Work out the finished part from the listing and answer in its coordinate system (mm). A direction names the side the tool comes from. Coordinates: 2 decimals unless noted, no trailing zeros. Order: outer loops, then holes, each group sorted by start corner. A loop starts at its lowest first (then second) coordinate and runs counter-clockwise, first axis right, second up.
1. A tool of negligible diameter and unlimited length cuts with its end or side. For faces 4 (the flat face through (29, 10.922, 2)), 5 (the flat face through (1.868, 3.297, -0.626)), 6 (the cylindrical face through (-24.159, 2.352, -3.858)), 7 (the flat face through (-19.553, 13.426, 4.948)), 8 (the flat face through (2.5, -4.4, 1.7)), from which of +Z, -Z, +X, -X, +Y, -Y can it reach the whole face along a straight path? Write none if from no direction.
2. The part is cut by section C-C, the plane y = 9.75. Give the vertices of the cut face in (x, z).
3. The part is cut by section B-B, the plane z = 1.75. Give the vertices of the cut face in (x, y).
4. The part is cut by section A-A, the plane y = 1.25. Give the vertices of the cut face in (x, z).
5. Determine the mould class of faces 1 (the flat face through (-5.059, 0, 2)), 2 (the flat face through (-1, 16.002, -1)), 3 (the cylindrical face through (-29.829, 13.498, 4.465)) for opening direction X: +X half, -X half, draft (parallel to the pull), parting line (faces both ways), or undercut.
6. Flat-ended cylindrical pins translate along their axes: pin 1 Ø12 at (x, y) = (17, 8) entering from -Z; pin 2 Ø5 at (x, z) = (1, -2) entering from +Y; pin 3 Ø4 at (x, z) = (-23, -6.5) entering from -Y; pin 4 Ø2 at (y, z) = (3, -4) entering from -X. Find the tip coordinate at first contact, or state that the pin passes through.
7. Find the intervals of material crossed by probe 1 along Y at (x, z) = (35, 1.25); probe 2 along X at (y, z) = (10.25, -6.75); probe 3 along Z at (x, y) = (-2.5, -4), in increasing order.
8. The part is cut by section D-D, the plane z = -2.75. Give the vertices of the cut face in (x, y).
```python
from build123d import *

# Parameters (mm, degrees)
SKETCH1_W                    = 25.4
SKETCH1_H                    = 21.844
BOLT_SIZE_WIDTH_HEIGHT_DEPTH = 7.62
FRONT_CURVE_DEPTH            = 22.844
SKETCH3_W                    = 25.4
SKETCH3_H                    = 21.844
REAR_CAP_DEPTH               = 1.27
WINGS_DEPTH                  = 21.844
HOOK_DEPTH_DEPTH             = 5.08
HOOK_HEIGHT_DEPTH            = 3.81
NUT_FLANGE_CLEARANCE_R       = 1.27
DECORATION_SIZE              = 2.54
CUT_EXTRUDE1_DEPTH           = 27.9240001


with BuildPart() as part:
    # Sketch1 → Bolt Size, Width, &Height (new body)
    with BuildSketch(Plane.XY):
        Rectangle(SKETCH1_W, SKETCH1_H)
        Polygon((0, 5.842), (-5.059320409, 2.921), (-5.059320409, -2.921), (0, -5.842), (5.059320409, -2.921), (5.059320409, 2.921), align=None, mode=Mode.SUBTRACT)
    extrude(amount=BOLT_SIZE_WIDTH_HEIGHT_DEPTH)

    # Sketch2 → Front Curve (cut, through all)
    with BuildSketch(Plane(origin=(0, 10.922, 0), x_dir=(1, 0, 0), z_dir=(0, 1, 0))):
        with BuildLine():
            Line((12.7, -7.62), (12.7, -3.81))
            ThreePointArc((12.7, -3.81), (0, -4.721818976), (-12.7, -3.81))
            Line((-12.7, -3.81), (-12.7, -7.62))
            Line((-12.7, -7.62), (12.7, -7.62))
        make_face()
    extrude(amount=-FRONT_CURVE_DEPTH, mode=Mode.SUBTRACT)

    # Sketch3 → Rear Cap (add)
    with BuildSketch(Plane(origin=(0, 0, 0), x_dir=(-1, 0, 0), z_dir=(0, 0, -1))):
        Rectangle(SKETCH3_W, SKETCH3_H)
        Polygon((-3.789320409, 2.187765158), (-3.789320409, -2.187765158), (0, -4.375530316), (3.789320409, -2.187765158), (3.789320409, 2.187765158), (0, 4.375530316), align=None, mode=Mode.SUBTRACT)
    extrude(amount=REAR_CAP_DEPTH)

    # Sketch6 → Wings (add)
    with BuildSketch(Plane.XZ.offset(10.922)):
        with BuildLine():
            ThreePointArc((-12.7, 3.81), (-25.407517395, 1.013767303), (-37.570763469, -3.607418757))
            Line((-37.570763469, -3.607418757), (-35.447209633, -8.161394654))
            ThreePointArc((-35.447209633, -8.161394654), (-24.318948968, -3.905861998), (-12.7, -1.27))
            Line((-12.7, -1.27), (-12.7, 3.81))
        make_face()
        with BuildLine():
            ThreePointArc((37.570763469, -3.607418757), (25.407517395, 1.013767303), (12.7, 3.81))
            Line((12.7, 3.81), (12.7, -1.27))
            ThreePointArc((12.7, -1.27), (24.318948968, -3.905861998), (35.447209633, -8.161394654))
            Line((35.447209633, -8.161394654), (37.570763469, -3.607418757))
        make_face()
    extrude(amount=-WINGS_DEPTH)

    # Sketch7 → Hook Depth (add)
    with BuildSketch(Plane(origin=(0, 10.922, 0), x_dir=(1, 0, 0), z_dir=(0, 1, 0))):
        with BuildLine():
            Line((12.7, 1.27), (-12.7, 1.27))
            ThreePointArc((-12.7, 1.27), (-24.318948968, 3.905861998), (-35.447209633, 8.161394654))
            Line((-35.447209633, 8.161394654), (-40.59977148, -2.888309885))
            ThreePointArc((-40.59977148, -2.888309885), (-30.779461435, -6.824786165), (-20.585837904, -9.657518799))
            Line((-20.585837904, -9.657518799), (-19.05, -2.656762978))
            ThreePointArc((-19.05, -2.656762978), (0, -4.721818976), (19.05, -2.656762978))
            Line((19.05, -2.656762978), (20.585837904, -9.657518799))
            ThreePointArc((20.585837904, -9.657518799), (30.779461435, -6.824786165), (40.59977148, -2.888309885))
            Line((40.59977148, -2.888309885), (35.447209633, 8.161394654))
            ThreePointArc((35.447209633, 8.161394654), (24.318948968, 3.905861998), (12.7, 1.27))
        make_face()
    extrude(amount=HOOK_DEPTH_DEPTH)

    # Sketch8 → Hook Height (add)
    with BuildSketch(Plane.XZ.offset(-10.922)):
        with BuildLine():
            ThreePointArc((-20.585837904, 9.657518799), (-30.779461435, 6.824786165), (-40.59977148, 2.888309885))
            Line((-40.59977148, 2.888309885), (-39.526321095, 0.586288106))
            ThreePointArc((-39.526321095, 0.586288106), (-29.965658216, 4.418684687), (-20.04155219, 7.176520399))
            Line((-20.04155219, 7.176520399), (-20.585837904, 9.657518799))
        make_face()
        with BuildLine():
            Line((39.526321095, 0.586288106), (40.59977148, 2.888309885))
            ThreePointArc((40.59977148, 2.888309885), (30.779461435, 6.824786165), (20.585837904, 9.657518799))
            Line((20.585837904, 9.657518799), (20.04155219, 7.176520399))
            ThreePointArc((20.04155219, 7.176520399), (29.965658216, 4.418684687), (39.526321095, 0.586288106))
        make_face()
    extrude(amount=HOOK_HEIGHT_DEPTH)

    # Nut Flange Clearance
    nut_flange_clearance_edges = [part.edges().sort_by_distance(p)[0] for p in [
        (5.059320409, 0, 4.577738649),
        (2.530429584, 4.381055799, 4.685798889),
        (-2.530429584, 4.381055799, 4.685798889),
        (-5.059320409, 0, 4.577738649),
        (-2.530429584, -4.381055799, 4.685798889),
        (2.530429584, -4.381055799, 4.685798889),
    ]]
    fillet(nut_flange_clearance_edges, radius=NUT_FLANGE_CLEARANCE_R)

    # Decoration
    decoration_edges = [part.edges().sort_by_distance(p)[0] for p in [
        (-40.063046287, 7.112, 1.737298996),
        (-20.313695047, 7.112, 8.417019599),
        (40.063046287, 7.112, 1.737298996),
        (20.313695047, 7.112, 8.417019599),
    ]]
    chamfer(decoration_edges, length=DECORATION_SIZE)

    # Sketch9 → Cut-Extrude1 (cut, through all)
    with BuildSketch(Plane(origin=(0, 16.002, 0), x_dir=(1, 0, 0), z_dir=(0, 1, 0))):
        with BuildLine():
            Line((40.59977148, -2.888309885), (39.526321095, -0.586288106))
            ThreePointArc((39.526321095, -0.586288106), (0, -9.349062527), (-39.526321095, -0.586288106))
            Line((-39.526321095, -0.586288106), (-40.59977148, -2.888309885))
            ThreePointArc((-40.59977148, -2.888309885), (0, -11.889062527), (40.59977148, -2.888309885))
        make_face()
    extrude(amount=-CUT_EXTRUDE1_DEPTH, mode=Mode.SUBTRACT)


solid = part.part
```
Geometry says:
1. face 4: +Z, +X, -Y
1. face 5: +Z, -Z
1. face 6: -Z, +Y, -Y
1. face 7: +Z, +Y, -Y
1. face 8: +Z
2. outline: (-37.57, -3.61) - (-35.45, -8.16) arc R83.88 cw to (-12.7, -1.27) - (12.7, -1.27) arc R83.88 cw to (35.45, -8.16) - (37.57, -3.61) arc R88.9 ccw to start
3. outline: (-36.93, 10.92) - (-22.79, 10.92) - (-22.79, -10.92) - (22.79, -10.92) - (22.79, 10.92) - (36.93, 10.92) - (36.93, 16) - (-36.93, 16) - close; hole (-5.06, -2.92) - (0, -5.84) - (5.06, -2.92) - (5.06, 2.92) - (0, 5.84) - (-5.06, 2.92) - close
4. outline: (-37.57, -3.61) - (-35.45, -8.16) arc R83.88 cw to (-12.7, -1.27) - (-3.79, -1.27) - (-3.79, 0) - (-5.06, 0) - (-5.06, 3.22) arc R1.27 ccw to (-6.42, 4.49) arc R88.9 ccw to start; (3.79, -1.27) - (12.7, -1.27) arc R83.88 cw to (35.45, -8.16) - (37.57, -3.61) arc R88.9 ccw to (6.42, 4.49) arc R1.27 ccw to (5.06, 3.22) - (5.06, 0) - (3.79, 0) - close
5. face 1: undercut
5. face 2: draft
5. face 3: -X half
6. pin 1: stops at z = -3.52
6. pin 2: stops at y = 16
6. pin 3: passes through
6. pin 4: stops at x = -37.57
7. probe 1: y = 10.92 to 16
7. probe 2: x = -36.11 to -32.25, 32.25 to 36.11
7. probe 3: z = -1.27 to 0
8. outline: (-37.97, 10.92) - (-35.67, 10.92) - (-35.67, -10.92) - (-20.11, -10.92) - (-20.11, 16) - (-37.97, 16) - close; (20.11, -10.92) - (35.67, -10.92) - (35.67, 10.92) - (37.97, 10.92) - (37.97, 16) - (20.11, 16) - close
